Here's how the part is built. I have some questions about the finished solid (model axes, mm). Round coordinates to 2 decimals unless told otherwise and drop trailing zeros. Loops run counter-clockwise (first coordinate to the right, second up) from the corner with the lowest first, then second, coordinate; pieces in that order, holes last. Notation, with made-up numbers: (-27, 53) -> (-18, 53) arc R8 cw to (-18, 58) -> close; hole circle Ø10 at (85, 57). An arc over 180 degrees is marked (long way). Use one line per item in the form item = value. Start each with the question number.
Item 1: If I drill on L1, parallel to Z at x = -36.5, y = 5.75; L2, parallel to X at y = -6.25, z = 21.5; L3, parallel to Z at x = -38, y = 13.5, over which ranges is the centre line in solid material (lowest first)? Write a range as [from, to].
Item 2: If we section it at B-B (y = 1.5): Write out the boundary of the cut face in (x, z), then the cut area to 4 significant figures.
Item 3: If we section it at A-A (x = -40): Write out the boundary of the cut face in (y, z).
Item 4: I'm going to push a flat-ended pin straight in: pin 1 Ø8 at (y, z) = (6, 30.5) entering from +X. Where does the tip first touch, or does it pass through?
Item 5: If we section it at C-C (z = 22): Write out the boundary of the cut face in (x, y).
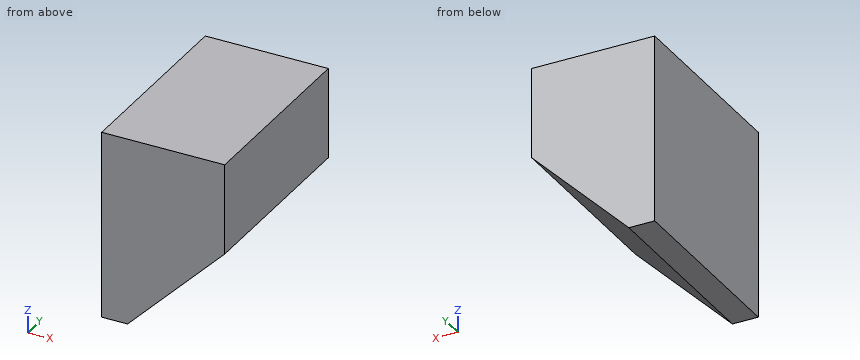
```python
from build123d import *

# Parameters (mm, degrees)
BOX112015002017004005_W     = 19
BOX112015002017004005_H     = 30
BOX112015002017004005_DEPTH = 29
CHAMFER005_SIZE             = 15


with BuildPart() as chamfer005:
    # Box112015002017004005 → Box112015002017004005 (new body)
    with BuildSketch(Plane(origin=(-47, -15, -15), x_dir=(1, 0, 0), z_dir=(0, 0, 1))):
        with Locations((9.5, 15)):
            Rectangle(BOX112015002017004005_W, BOX112015002017004005_H)
    extrude(amount=BOX112015002017004005_DEPTH)

    # Chamfer005
    chamfer005_edges = [chamfer005.edges().sort_by_distance(p)[0] for p in [
        (-28, 0, 14),
    ]]
    chamfer(chamfer005_edges, length=CHAMFER005_SIZE)


with BuildPart() as chamfer005_1:
    # Chamfer005 placement: moved
    add(chamfer005.part.moved(Location((0, 0, 6))))


with BuildPart() as part_mirroring005:
    # Part__Mirroring005: instance of Chamfer005
    add(chamfer005_1.part.mirror(Plane(origin=(0, 0, 20), x_dir=(0, 1, 0), z_dir=(0, 0, 1))))


solid = part_mirroring005.part
```
Values found:
q1.L1 = [26.5, 49]
q1.L2 = [-47, -41.5]
q1.L3 = [25, 49]
q2.outline = (-47, 20) -> (-43, 20) -> (-28, 35) -> (-28, 49) -> (-47, 49) -> close
q2.area = 438.5 mm2
q3.outline = (-15, 23) -> (15, 23) -> (15, 49) -> (-15, 49) -> close
q4.pin_1 = -28.5
q5.outline = (-47, -15) -> (-41, -15) -> (-41, 15) -> (-47, 15) -> close
